Autodesk Inventor part; units mm, degrees
ref_plane "YZ Plane" through (0, 0, 0) normal (1, 0, 0) x (0, 1, 0)
ref_plane "XZ Plane" through (0, 0, 0) normal (0, 1, 0) x (-1, 0, 0)
ref_plane "XY Plane" through (0, 0, 0) normal (0, 0, 1) x (1, 0, 0)
sketch "Sketch1" plane through (0, 0, 0) normal (0, 1, 0) x (-1, 0, 0)
  line L0 (0, 0) -> (30.7, 0)
  line L1 (30.7, 0) -> (30.7, 30.7)
  line L2 (30.7, 30.7) -> (0, 30.7)
  line L3 (0, 30.7) -> (0, 0)
  dimension "d0" = 30.7
  dimension "d1" = 30.7
extrude "Extrusion1" add sketch "Sketch1" along normal blind 2.032
sketch "Sketch2" plane through (0, 2.032, 0) normal (0, 1, 0) x (1, 0, 0)
  circle A0 centre (-26.89, -26.89) radius 3.81
  circle A1 centre (-3.81, -26.89) radius 3.81
  circle A2 centre (-3.81, -3.81) radius 3.81
  circle A3 centre (-26.89, -3.81) radius 3.81
  circle A4 centre (-15.35, -30.9598) radius 7.2278
  circle A5 centre (-15.35, 0.2598) radius 7.2278
  circle A6 centre (-30.9598, -15.35) radius 7.2278
  circle A7 centre (0.2598, -15.35) radius 7.2278
  line L0 (-29.5841, -24.1959) -> (-25.849, -20.4608)
  line L1 (-25.849, -10.2392) -> (-29.5841, -6.5041)
  line L2 (-24.1959, -1.1159) -> (-20.4608, -4.851)
  line L3 (-10.2392, -4.851) -> (-6.5041, -1.1159)
  line L4 (-1.1159, -6.5041) -> (-4.851, -10.2392)
  line L5 (-4.851, -20.4608) -> (-1.1159, -24.1959)
  line L6 (-6.5041, -29.5841) -> (-10.2392, -25.849)
  line L7 (-20.4608, -25.849) -> (-24.1959, -29.5841)
  line L8 (-30.7, 0) -> (-30.7, -30.7)
  line L9 (-30.7, -30.7) -> (0, -30.7)
  line L10 (0, -30.7) -> (0, 0)
  line L11 (0, 0) -> (-30.7, 0)
  line L12 (-23.732, -15.35) -> (-6.968, -15.35) construction
  line L13 (-30.7, -15.35) -> (-23.732, -15.35) construction
  point P0 (-26.89, 0)
  point P1 (-3.81, 0)
  point P2 (-30.7, -3.81)
  point P3 (0, -3.81)
  point P4 (0, -26.89)
  point P5 (-3.81, -30.7)
  point P6 (-26.89, -30.7)
  point P7 (-30.7, -26.89)
  dimension "d4" = 7.62
  dimension "d5" = 16.764
extrude "Extrusion2" cut sketch "Sketch2" against normal through all contours A0 L8 A6 L0 | L7 A4 L9 A0 | A0 L9 L8 | A6 L8 | A4 L9 | L6 A1 L9 A4 | L8 A3 L1 A6 | L8 L11 A3 | A1 L10 L9 | L5 A7 L10 A1 | L11 A5 L2 A3 | A7 L10 | L11 A5 | L4 A2 L10 A7 | L11 A2 L3 A5 | L11 L10 A2 picked at (-27.8979, -13.6464) picked at (-16.0496, -27.92) picked at (-4.1409, -17.2716) picked at (-14.1643, -2.5459)
sketch "Sketch3" plane through (0, 2.032, 0) normal (0, 1, 0) x (1, 0, 0)
  circle A0 centre (-26.89, -26.89) radius 1.524
  circle A1 centre (-21.8611, -21.8611) radius 1.524
  circle A2 centre (-15.35, -15.35) radius 4.826
  arc A3 (-29.5841, -24.1959) -> (-24.1959, -29.5841) centre (-26.89, -26.89) ccw
  line L0 (-29.5841, -29.5841) -> (0, 0) construction
  line L1 (-25.4985, -30.4368) -> (-30.4368, -25.4985) construction
  line L2 (-18.0893, -23.4775) -> (-23.4775, -18.0893) construction
  arc A4 (-29.5841, -24.1959) -> (-24.1959, -29.5841) centre (-26.89, -26.89) ccw
  line L3 (-24.1959, -29.5841) -> (-20.4608, -25.849)
  arc A5 (-10.2392, -25.849) -> (-20.4608, -25.849) centre (-15.35, -30.9598) ccw
  line L4 (-10.2392, -25.849) -> (-6.5041, -29.5841)
  arc A6 (-6.5041, -29.5841) -> (-1.1159, -24.1959) centre (-3.81, -26.89) ccw
  line L5 (-1.1159, -24.1959) -> (-4.851, -20.4608)
  arc A7 (-4.851, -10.2392) -> (-4.851, -20.4608) centre (0.2598, -15.35) ccw
  line L6 (-4.851, -10.2392) -> (-1.1159, -6.5041)
  arc A8 (-1.1159, -6.5041) -> (-6.5041, -1.1159) centre (-3.81, -3.81) ccw
  line L7 (-6.5041, -1.1159) -> (-10.2392, -4.851)
  arc A9 (-20.4608, -4.851) -> (-10.2392, -4.851) centre (-15.35, 0.2598) ccw
  line L8 (-20.4608, -4.851) -> (-24.1959, -1.1159)
  arc A10 (-24.1959, -1.1159) -> (-29.5841, -6.5041) centre (-26.89, -3.81) ccw
  line L9 (-29.5841, -6.5041) -> (-25.849, -10.2392)
  arc A11 (-25.849, -20.4608) -> (-25.849, -10.2392) centre (-30.9598, -15.35) ccw
  line L10 (-25.849, -20.4608) -> (-29.5841, -24.1959)
  line L11 (-29.5841, -1.1159) -> (-1.1159, -29.5841) construction
  circle A12 centre (-3.81, -26.89) radius 1.524
  circle A13 centre (-8.8389, -21.8611) radius 1.524
  circle A14 centre (-3.81, -3.81) radius 1.524
  circle A15 centre (-8.8389, -8.8389) radius 1.524
  circle A16 centre (-26.89, -3.81) radius 1.524
  circle A17 centre (-21.8611, -8.8389) radius 1.524
  dimension "d8" = 3.048
  dimension "d9" = 3.048
  dimension "d10" = 10.16
  dimension "d11" = 9.652
  dimension "d14" = 360
extrude "Extrusion3" cut sketch "Sketch3" against normal through all contours A0 | A1 | A2 | A12 | A13 | A14 | A15 | A16 | A17
properties part number "Brushless Motor Mount"
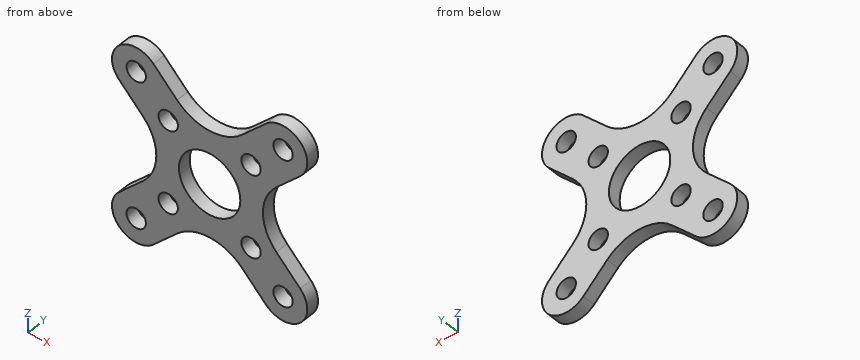
Can you work these out from the model? Positions are in its coordinate system, mm. Round coordinates to 2 decimals unless told otherwise and drop trailing zeros. Order: outer loops, then holes, each group sorted by start corner. A loop starts at its lowest first (then second) coordinate and runs counter-clockwise, first axis right, second up. Notation, with made-up numbers: (62, -15) -> (78, -15) arc R24 cw to (78, -2) -> close; hole circle Ø5 at (60.5, 4). An arc over 180 degrees is marked (long way). Return JSON: item names as keys, results as strings. Group by question number.
1. If we section it at D-D, the plane z = 3.81: Write out the boundary of the cut face in (x, y), then the cut area to 3 significant figures.
2. If we section it at C-C, the plane x = -8: Write out the boundary of the cut face in (y, z), then the cut area to 3 significant figures.
3. If we section it at A-A, the plane x = -15.35: Write out the boundary of the cut face in (y, z), then the cut area to 3 significant figures.
4. If we section it at B-B, the plane z = 15.35: Write out the boundary of the cut face in (x, y), then the cut area to 3 significant figures.
5. I need wall thicknesses on line 1 (Z direction, x = -9.5, y = 1.25); line 2 (Z direction, x = -10, y = 0.35); line 3 (Z direction, x = -3.81, y = 1.5). Which ranges of each line are inside material? Lowest first, please. Write a range as [from, to].
6. Will this pin go through, and if not, where does the flat tip stop? pin 1 (5 mm diameter, centred on x = -3.81, z = 26.89, fed in from +Y).
Output values:
{
 "1": {"outline": "(-30.7, 0) -> (-28.41, 0) -> (-28.41, 2.03) -> (-30.7, 2.03) -> close; (-25.37, 0) -> (-21.5, 0) -> (-21.5, 2.03) -> (-25.37, 2.03) -> close; (-9.2, 0) -> (-5.33, 0) -> (-5.33, 2.03) -> (-9.2, 2.03) -> close; (-2.29, 0) -> (0, 0) -> (0, 2.03) -> (-2.29, 2.03) -> close", "area": "25.0 mm²"},
 "2": {"outline": "(0, 2.61) -> (2.03, 2.61) -> (2.03, 7.57) -> (0, 7.57) -> close; (0, 10.11) -> (2.03, 10.11) -> (2.03, 20.59) -> (0, 20.59) -> close; (0, 23.13) -> (2.03, 23.13) -> (2.03, 28.09) -> (0, 28.09) -> close", "area": "41.4 mm²"},
 "3": {"outline": "(0, 6.97) -> (2.03, 6.97) -> (2.03, 10.52) -> (0, 10.52) -> close; (0, 20.18) -> (2.03, 20.18) -> (2.03, 23.73) -> (0, 23.73) -> close", "area": "14.5 mm²"},
 "4": {"outline": "(-23.73, 0) -> (-20.18, 0) -> (-20.18, 2.03) -> (-23.73, 2.03) -> close; (-10.52, 0) -> (-6.97, 0) -> (-6.97, 2.03) -> (-10.52, 2.03) -> close", "area": "14.5 mm²"},
 "5": {"line 1": "[4.11, 7.47], [10.21, 20.49], [23.23, 26.59]", "line 2": "[4.61, 7.85], [9.83, 20.87], [22.85, 26.09]", "line 3": "[0, 2.29], [5.33, 9.2], [21.5, 25.37], [28.41, 30.7]"},
 "6": {"pin 1": "y = 2.03"}
}
